The listing builds one solid part. Answer for the finished solid, in the listing's coordinates (mm). Face numbers are marked on the shaded views. A direction names the side the tool comes from. Round coordinates to 2 decimals unless told otherwise and drop trailing zeros. Loops run counter-clockwise (first coordinate to the right, second up) from the corner with the lowest first, then second, coordinate; pieces in that order, holes last. Notation, with made-up numbers: M 1,6 L 36,6 A22 cw 36,45 Z; hole C 81,69 d8. An arc over 180 degrees is marked long. Put each result on its own line as item: value. Start each with the question number.
(1) Straight lines are drawn through the part: line 1 (Z direction, x = -3.25, y = -1.75); line 2 (Y direction, x = -0.25, z = -2); line 3 (X direction, y = 2.25, z = -2.5). For each, find the intervals that lie inside material, in ascending order.
(2) Section A-A, the plane x = 0 is taken. Determine the outline of the cut face in (y, z).
(3) Section C-C, the plane z = -4.5 is taken. Determine the outline of the cut face in (x, y), then the cut area to 3 significant figures.
(4) Section D-D, the plane x = -4.5 is taken. Determine the outline of the cut face in (y, z).
(5) A flat-ended cylindrical pin translates along its axis: P1, Ø5, axis at x = -2.5, y = -3.5, coming from the +Z side. Find the tip coordinate at first contact, or state that the pin passes through.
(6) Determine the mould class of the marked faces 1, 2 and 3 for opening direction X: released by +X, released by -X, zero draft, split by the parting line, or undercut.
(7) Which of the six approach directions +Z, -Z, +X, -X, +Y, -Y give full straight-line access (tool end or side, diameter ignored) to the marked faces 4 and 5?
(8) Section B-B, the plane y = 0 is taken. Determine the outline of the cut face in (x, z), then the cut area to 3 significant figures.
```python
from build123d import *

# Parameters (mm, degrees)
BOX010_W          = 13.4
BOX010_H          = 12.5
BOX010_DEPTH      = 6.6
CYLINDER002_R     = 3.3
CYLINDER002_DEPTH = 5


with BuildPart() as rotary_base:
    # Box010 → Box010 (new body)
    with BuildSketch(Plane(origin=(-6.7, -6.25, -11.6), x_dir=(1, 0, 0), z_dir=(0, 0, 1))):
        with Locations((6.7, 6.25)):
            Rectangle(BOX010_W, BOX010_H)
    extrude(amount=BOX010_DEPTH)


with BuildPart() as fusion020:
    # Cylinder002 → Cylinder002 (new body)
    with BuildSketch(Plane.XY.offset(-5)):
        Circle(CYLINDER002_R)
    extrude(amount=CYLINDER002_DEPTH)

    # Fusion020: union ROTARY_base
    add(rotary_base.part)


solid = fusion020.part
```
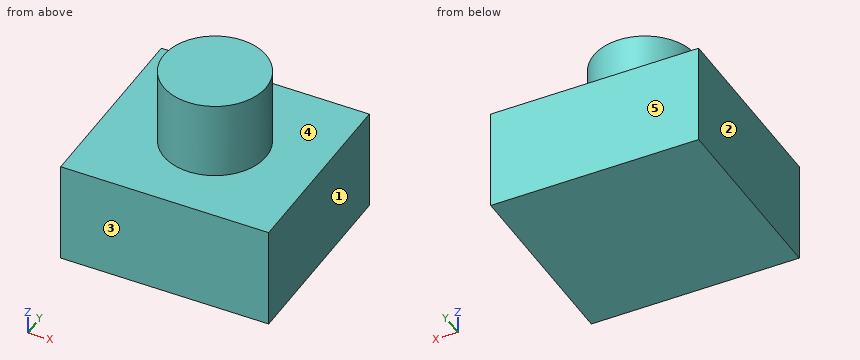
Recorded:
1. line 1: z = -11.6 to -5
1. line 2: y = -3.29 to 3.29
1. line 3: x = -2.41 to 2.41
2. outline: M -6.25,-11.6 L 6.25,-11.6 L 6.25,-5 L 3.3,-5 L 3.3,0 L -3.3,0 L -3.3,-5 L -6.25,-5 Z
3. outline: C 0,0 d6.6
3. area: 34.2 mm²
4. outline: M -6.25,-11.6 L 6.25,-11.6 L 6.25,-5 L -6.25,-5 Z
5. P1: stops at z = 0
6. face 1: released by +X
6. face 2: released by -X
6. face 3: zero draft
7. face 4: +Z
7. face 5: +Z, -Z, +X, -X, +Y
8. outline: M -6.7,-11.6 L 6.7,-11.6 L 6.7,-5 L 3.3,-5 L 3.3,0 L -3.3,0 L -3.3,-5 L -6.7,-5 Z
8. area: 121 mm²
